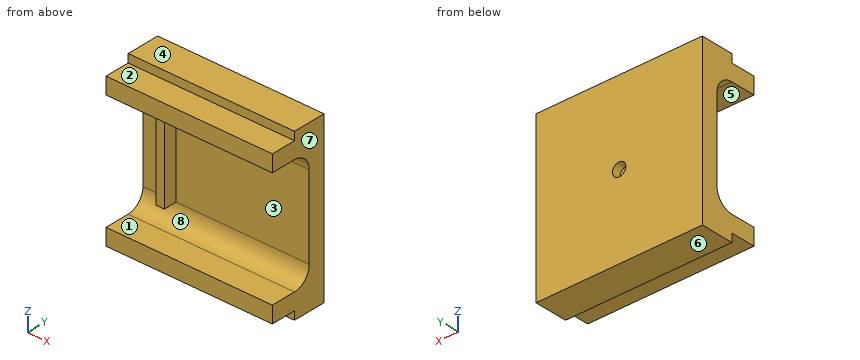
```python
from build123d import *

# Parameters (mm, degrees)
SKETCH1_W           = 100
SKETCH1_H           = 100
BOSS_EXTRUDE1_DEPTH = 20
SKETCH3_R           = 4
CUT_EXTRUDE1_DEPTH  = 5
SKETCH4_W           = 100
SKETCH4_H           = 10
BOSS_EXTRUDE2_DEPTH = 15
SKETCH5_W           = 100
SKETCH5_H           = 70
CUT_EXTRUDE2_DEPTH  = 10
FILLET2_R           = 10
FILLET3_R           = 10
SKETCH6_W           = 5
SKETCH6_H           = 50
BOSS_EXTRUDE3_DEPTH = 8


with BuildPart() as part:
    # Sketch1 → Boss-Extrude1 (new body)
    with BuildSketch(Plane(origin=(0, 0, 0), x_dir=(1, 0, 0), z_dir=(0, 1, 0))):
        Rectangle(SKETCH1_W, SKETCH1_H)
    extrude(amount=BOSS_EXTRUDE1_DEPTH)

    # Sketch3 → Cut-Extrude1 (cut)
    with BuildSketch(Plane(origin=(0, 20, 0), x_dir=(1, 0, 0), z_dir=(0, 1, 0))):
        with Locations(Location((0, 0, 0), (0, 0, 270))):
            Circle(SKETCH3_R)
    extrude(amount=-CUT_EXTRUDE1_DEPTH, mode=Mode.SUBTRACT)

    # Sketch4 → Boss-Extrude2 (add)
    with BuildSketch(Plane.XZ):
        with Locations((0, -40)):
            Rectangle(SKETCH4_W, SKETCH4_H)
        with Locations((0, 40)):
            Rectangle(SKETCH4_W, SKETCH4_H)
    extrude(amount=BOSS_EXTRUDE2_DEPTH)

    # Sketch5 → Cut-Extrude2 (cut)
    with BuildSketch(Plane.XZ):
        Rectangle(SKETCH5_W, SKETCH5_H)
    extrude(amount=-CUT_EXTRUDE2_DEPTH, mode=Mode.SUBTRACT)

    # Fillet2
    fillet2_edges = [part.edges().sort_by_distance(p)[0] for p in [
        (0, 10, -35),
    ]]
    fillet(fillet2_edges, radius=FILLET2_R)

    # Fillet3
    fillet3_edges = [part.edges().sort_by_distance(p)[0] for p in [
        (0, 10, 35),
    ]]
    fillet(fillet3_edges, radius=FILLET3_R)

    # Sketch6 → Boss-Extrude3 (add)
    with BuildSketch(Plane.XZ.offset(-10)):
        with Locations((-32.5, 0)):
            Rectangle(SKETCH6_W, SKETCH6_H)
    extrude(amount=BOSS_EXTRUDE3_DEPTH)


solid = part.part
```
Check sheet for the modelled part. Datum: model origin and axes. Units: mm. Face numbers are marked on the shaded views. A direction names the side the tool comes from. Coordinates: 2 decimals unless noted, no trailing zeros. Loops run counter-clockwise (first coordinate to the right, second up) from the corner with the lowest first, then second, coordinate; pieces in that order, holes last.
1) Sectioned sample at C-C (y = 7.5). Record the boundary of the cut face in (x, z), and give its area (3 significant figures).
2) Sectioned sample at D-D (x = 0). Record the boundary of the cut face in (y, z).
3) Access from +Z, -Z, +X, -X, +Y, -Y to the whole of each face (thin tool, end or side, straight path). Record for the marked faces 1, 2, 3 and 4.
4) Material ranges on probe 1 along Z at (x, y) = (-21, -1); probe 2 along X at (y, z) = (18.8, 0); probe 3 along Y at (x, z) = (11, 15), recorded low to high.
5) Sectioned sample at B-B (z = -10.5). Record the boundary of the cut face in (x, y).
6) Gauge pin test, flat ends, axial feed: pin 1 (8 mm diameter, centred on x = 22, z = 27, fed in from -Y); pin 2 (8 mm diameter, centred on x = -27.5, z = 17, fed in from -Y); pin 3 (1.5 mm diameter, centred on x = -3.5, z = -20, fed in from -Y). Record the tip position at first contact, or that the pin passes through.
7) Release check for a two-part mould opening along Z. For the marked faces 5, 6, 7 and 8 record: released by +Z, released by -Z, zero draft, split by the parting line, or undercut.
8) Sectioned sample at A-A (y = -1.5). Record the boundary of the cut face in (x, z).
Check sheet entries:
1. outline: (-50, -50) - (50, -50) - (50, -31.61) - (-50, -31.61) - close; (-50, 31.61) - (50, 31.61) - (50, 50) - (-50, 50) - close; (-35, -25) - (-30, -25) - (-30, 25) - (-35, 25) - close
1. area: 3,930 mm2
2. outline: (-15, -45) - (0, -45) - (0, -50) - (20, -50) - (20, -4) - (15, -4) - (15, 4) - (20, 4) - (20, 50) - (0, 50) - (0, 45) - (-15, 45) - (-15, 35) - (0, 35) arc R10 cw to (10, 25) - (10, -25) arc R10 cw to (0, -35) - (-15, -35) - close
3. face 1: +X, -X, -Y
3. face 2: +Z, +X, -X, -Y
3. face 3: +X, -Y
3. face 4: +Z, +X, -X, +Y, -Y
4. probe 1: z = -45 to -35, 35 to 45
4. probe 2: x = -50 to -4, 4 to 50
4. probe 3: y = 10 to 20
5. outline: (-50, 10) - (-35, 10) - (-35, 2) - (-30, 2) - (-30, 10) - (50, 10) - (50, 20) - (-50, 20) - close
6. pin 1: stops at y = 8
6. pin 2: stops at y = 2
6. pin 3: stops at y = 10
7. face 5: undercut
7. face 6: released by -Z
7. face 7: zero draft
7. face 8: undercut
8. outline: (-50, -45) - (50, -45) - (50, -35) - (-50, -35) - close; (-50, 35) - (50, 35) - (50, 45) - (-50, 45) - close
